Input: part model. Units: mm. Frame: model coordinates. A direction names the side the tool comes from. Round coordinates to 2 decimals unless told otherwise and drop trailing zeros. Loops run counter-clockwise (first coordinate to the right, second up) from the corner with the lowest first, then second, coordinate; pieces in that order, holes last.
(1) Access query for faces 4 (the face through (33.927, -19.72, 5.867)), 5 (the face through (24.56, 1.48, 3.68)), 6 (the face through (0.224, 1.479, -0.045)). Directions: +Z, -Z, +X, -X, +Y, -Y. A direction counts if a zero-diameter tool reaches every point of the face in a straight line with its end or side. Return the directions, or none.
(2) First-contact query: pin 1 Ø12 at (x, y) = (44.5, -26) entering from -Z; pin 2 Ø2.5 at (x, y) = (0.5, 2) entering from +Z; pin 3 Ø1.8 at (x, z) = (-0.8, 0) entering from +Y; pin 4 Ø2.5 at (x, z) = (-8.8, 0) entering from -Y. Flat tips, straight axial feed; report the tip coordinate or a pass-through.
(3) Cut plane B-B, the plane y = -39. Output: boundary loops of the cut face in (x, z), and give its area (3 significant figures).
(4) Line query: line 1 (Z direction, x = -8.8, y = 0.8) (3 decimals); line 2 (Y direction, x = 36, z = 6); line 3 (Z direction, x = -16, y = 2). Output: solid intervals per line, ascending.
(5) Draft query along Z for faces 1 (the face through (19.36, -41.48, 12.21)), 2 (the face through (64.673, -41.479, 34.262)), 3 (the face through (-15.776, 1.479, -0.045)). Return one class per face: released by +Z, released by -Z, zero draft, split by the parting line, or undercut.
(6) Cut plane C-C, the plane x = -8.8. Output: boundary loops of the cut face in (y, z) (3 decimals), and give its area (3 significant figures).
(7) Cut plane A-A, the plane x = 5. Output: boundary loops of the cut face in (y, z), and give its area (3 significant figures).
Autodesk Inventor part; units mm, degrees
ref_plane "YZ Plane" through (0, 0, 0) normal (1, 0, 0) x (0, 1, 0)
ref_plane "XZ Plane" through (0, 0, 0) normal (0, 1, 0) x (-1, 0, 0)
ref_plane "XY Plane" through (0, 0, 0) normal (0, 0, 1) x (1, 0, 0)
sketch "Sketch1" plane through (0, 0, 0) normal (0, 1, 0) x (-1, 0, 0)
  line L0 (-11.4129, 10) -> (10.3431, 10)
  line L1 (20, 2) -> (20, -2)
  line L2 (10.3431, -10) -> (-17.4129, -10)
  line L3 (-20, -10) -> (-20, 10)
  line L4 (20, -10) -> (-20, 10) construction
  line L5 (20, 10) -> (-20, -10) construction
  line L6 (13.1716, -8.8284) -> (17.6284, -4.3716)
  line L7 (13.1716, 8.8284) -> (17.6284, 4.3716)
  line L8 (18.8, 1.5431) -> (18.8, -1.5431)
  arc A0 (18.8, 1.5431) -> (17.6284, 4.3716) centre (14.8, 1.5431) ccw
  arc A1 (17.6284, -4.3716) -> (18.8, -1.5431) centre (14.8, -1.5431) ccw
  arc A2 (13.1716, 8.8284) -> (10.3431, 10) centre (10.3431, 6) ccw
  arc A3 (10.3431, -10) -> (13.1716, -8.8284) centre (10.3431, -6) ccw
  line L9 (-18, -10) -> (-12, 10)
  line L10 (-12.5623, 10.1687) -> (-26.3566, 14.307)
  line L11 (-33.8781, 16.5634) -> (-39.8781, -3.4366)
  line L12 (-35.8836, -4.6349) -> (-18.5623, -9.8313)
  line L13 (-26.8781, 14.4634) -> (-37.0046, -4.2986)
  line L14 (-27.3388, 14.7536) -> (-59.1142, 34.7654)
  line L15 (-37.7675, -3.4111) -> (-65.2661, 28.5779)
  arc A4 (-12.5623, 10.1687) -> (-11.4129, 10) centre (-11.4129, 14) ccw
  arc A5 (-18.5623, -9.8313) -> (-17.4129, -10) centre (-17.4129, -6) ccw
  arc A6 (-27.3388, 14.7536) -> (-26.3566, 14.307) centre (-25.2072, 18.1383) ccw
  arc A7 (-37.7675, -3.4111) -> (-35.8836, -4.6349) centre (-34.7342, -0.8036) ccw
  arc A8 (-59.1142, 34.7654) -> (-65.2661, 28.5779) centre (-61.5814, 31.0663) ccw
  line L16 (18.8, 0) -> (8.8, 0)
  circle A9 centre (0.8, 0) radius 1.025
  circle A10 centre (8.8, -8) radius 1.025
  circle A11 centre (16.8, 0) radius 1.025
  circle A12 centre (8.8, 8) radius 1.025
  line L17 (-23.0219, -4.861) -> (-29.7868, -2.8316)
  line L18 (-22.3993, -4.5258) -> (-18.4228, 8.7292)
  line L19 (-19.263, 9.2186) -> (-30.0044, -2.007)
  arc A13 (-23.0219, -4.861) -> (-22.3993, -4.5258) centre (-22.8782, -4.3821) ccw
  arc A14 (-30.0044, -2.007) -> (-29.7868, -2.8316) centre (-29.6432, -2.3526) ccw
  arc A15 (-18.4228, 8.7292) -> (-19.263, 9.2186) centre (-18.9017, 8.8729) ccw
  line L20 (-37.6066, 5.1132) -> (-33.634, 12.4734)
  line L21 (-33.634, 12.4734) -> (-55.2323, 26.0758)
  line L22 (-55.8779, 25.3268) -> (-38.4257, 5.0247)
  arc A16 (-38.4257, 5.0247) -> (-37.6066, 5.1132) centre (-38.0466, 5.3506) ccw
  arc A17 (-55.2323, 26.0758) -> (-55.8779, 25.3268) centre (-55.4988, 25.6528) ccw
  point P0 (0, 0)
  point P1 (0, 0)
  point P2 (12, -10)
  point P3 (12, 10)
  point P4 (20, 10)
  point P5 (18.8, 3.2)
  point P6 (18.8, -3.2)
  point P7 (-37.9518, 4.4734)
  point P8 (-35.6203, 8.7933)
  dimension "d0" = 40
  dimension "d1" = 20
  dimension "d32" = 8
  dimension "d33" = 8
  dimension "d34" = 8
  dimension "d35" = 8
  dimension "d43" = 1.2
  dimension "d46" = 4
  dimension "d47" = 2
  dimension "d48" = 8
  dimension "d49" = 3
  dimension "d50" = 7
  dimension "d51" = 43.3541
  dimension "d52" = 32.617
  dimension "d53" = 4
  dimension "d54" = 10
  dimension "d55" = 2.05
  dimension "d56" = 8
  dimension "d59" = 360
  dimension "d79" = 0.5
  dimension "d80" = 8
  dimension "d81" = 5
  dimension "d82" = 5
  dimension "d83" = 0.5
extrude "Extrusion1" add sketch "Sketch1" along normal blind 3
sketch "Sketch8" plane through (0, 0, 0) normal (0, -1, 0) x (1, 0, 0)
  arc A0 (17.4129, -10) -> (18.5623, -9.8313) centre (17.4129, -6) ccw
  line L0 (-13.1716, -8.8284) -> (-17.6284, -4.3716)
  arc A1 (35.8836, -4.6349) -> (37.7675, -3.4111) centre (34.7342, -0.8036) ccw
  circle A2 centre (34.7342, -0.8036) radius 1.5
  circle A3 centre (30.2342, 11.6964) radius 1.5
  line L1 (65.2661, 28.5779) -> (37.7675, -3.4111)
  line L2 (27.3388, 14.7536) -> (59.1142, 34.7654)
  line L3 (15.9075, -6.542) -> (11.4075, 5.958)
  line L4 (14.4183, 7.042) -> (18.9183, -5.458)
  arc A4 (15.9075, -6.542) -> (18.9183, -5.458) centre (17.4129, -6) ccw
  arc A5 (14.4183, 7.042) -> (11.4075, 5.958) centre (12.9129, 6.5) ccw
  line L5 (34.7342, -0.8036) -> (30.2342, 11.6964) construction
  line L6 (36.1456, -0.2955) -> (31.6456, 12.2045)
  line L7 (28.8229, 11.1883) -> (33.3229, -1.3117)
  arc A6 (33.3229, -1.3117) -> (36.1456, -0.2955) centre (34.7342, -0.8036) ccw
  arc A7 (31.6456, 12.2045) -> (28.8229, 11.1883) centre (30.2342, 11.6964) ccw
  line L8 (59.3782, 24.0575) -> (55.8591, 30.2331) construction
  line L9 (60.5121, 24.7036) -> (56.993, 30.8792)
  line L10 (54.7253, 29.587) -> (58.2444, 23.4114)
  arc A8 (58.2444, 23.4114) -> (60.5121, 24.7036) centre (59.3782, 24.0575) ccw
  arc A9 (56.993, 30.8792) -> (54.7253, 29.587) centre (55.8591, 30.2331) ccw
  point P0 (0, 0)
  point P1 (17.9938, -9.9576)
  point P2 (15.1629, 0.25)
  point P3 (32.4842, 5.4464)
  point P4 (57.6187, 27.1453)
  dimension "d64" = 3
  dimension "d69" = 3
  dimension "d70" = 4.5
  dimension "d71" = 12.5
  dimension "d88" = 1.6
extrude "Extrusion7" add sketch "Sketch8" along normal blind 40
extrude "Extrusion8" add sketch "Sketch1" against normal blind 3 from surface at -40 contours A11 L16 | L16 A11 | L0 A2 L7 A0 L8 A1 L6 A3 L2 A5 L12 A7 L15 A8 L14 A6 L10 A4 | A9 | A10 | A12
sketch "Sketch10" plane through (-10.3431, -43, -10) normal (0, -1, 0) x (1, 0, 0)
  line L0 (-8.4569, 8.4569) -> (-8.4569, 11.5431)
  line L1 (-8.4569, 10) -> (1.5431, 10)
  circle A0 centre (1.5431, 10) radius 1.5
  point P0 (10.3431, 10)
  dimension "d84" = 10
  dimension "d85" = 3
extrude "Extrusion9" cut sketch "Sketch10" against normal blind 3
properties part number "leg_part"
Reported:
1. face 4: +Z, +X
1. face 5: +Y, -Y
1. face 6: +Y
2. pin 1: passes through
2. pin 2: stops at z = 10
2. pin 3: stops at y = -40
2. pin 4: stops at y = 0
3. outline: (11.41, 5.96) - (15.91, -6.54) arc R1.6 ccw to (18.92, -5.46) - (14.42, 7.04) arc R1.6 ccw to start; (28.82, 11.19) - (33.32, -1.31) arc R1.5 ccw to (36.15, -0.3) - (31.65, 12.2) arc R1.5 ccw to start; (54.73, 29.59) - (58.24, 23.41) arc R1.31 ccw to (60.51, 24.7) - (56.99, 30.88) arc R1.31 ccw to start
3. area: 121 mm2
4. line 1: z = -10 to -9.025, -6.975 to 6.975, 9.025 to 10
4. line 2: y = -43 to -40, 0 to 3
4. line 3: z = -6 to -0.64, 0.64 to 6
5. face 1: released by +Z
5. face 2: split by the parting line
5. face 3: undercut
6. outline: (-43, -10) - (-40, -10) - (-40, -1.5) - (-43, -1.5) - close; (-43, 1.5) - (-40, 1.5) - (-40, 10) - (-43, 10) - close; (0, -10) - (3, -10) - (3, -9.025) - (0, -9.025) - close; (0, -6.975) - (3, -6.975) - (3, 6.975) - (0, 6.975) - close; (0, 9.025) - (3, 9.025) - (3, 10) - (0, 10) - close
6. area: 98.7 mm2
7. outline: (-43, -10) - (-40, -10) - (-40, 10) - (-43, 10) - close; (0, -10) - (3, -10) - (3, 10) - (0, 10) - close
7. area: 120 mm2
